Could you check a few things on this model? Use its own coordinates, in mm. Round coordinates to 2 decimals unless told otherwise and drop trailing zeros. Loops run counter-clockwise (first coordinate to the right, second up) from the corner with the lowest first, then second, coordinate; pieces in that order, holes last. Notation, with made-up numbers: (58.5, 5) - (99.5, 5) arc R23 ccw to (99.5, 34) - close; hole circle Ø6 at (-27, 67). An arc over 180 degrees is marked (long way). Use one line per item in the form item = value.
```python
from build123d import *

# Parameters (mm, degrees)
BOSS_EXTRUDE1_DEPTH = 1.5
SKETCH2_R           = 9
CUT_EXTRUDE3_DEPTH  = 1.5


with BuildPart() as part:
    # Sketch1 → Boss-Extrude1 (new body)
    with BuildSketch(Plane(origin=(0, 0, 0), x_dir=(1, 0, 0), z_dir=(0, 1, 0))):
        with BuildLine():
            Line((-97.5, 40), (97.5, 40))
            ThreePointArc((97.5, 40), (115.17766953, 32.67766953), (122.5, 15))
            Line((122.5, 15), (122.5, -15))
            ThreePointArc((122.5, -15), (115.17766953, -32.67766953), (97.5, -40))
            Line((97.5, -40), (-97.5, -40))
            ThreePointArc((-97.5, -40), (-115.17766953, -32.67766953), (-122.5, -15))
            Line((-122.5, -15), (-122.5, 15))
            ThreePointArc((-122.5, 15), (-115.17766953, 32.67766953), (-97.5, 40))
        make_face()
    extrude(amount=BOSS_EXTRUDE1_DEPTH)

    # Sketch2 → Cut-Extrude3 (cut)
    with BuildSketch(Plane(origin=(0, 1.5, 0), x_dir=(1, 0, 0), z_dir=(0, 1, 0))):
        with Locations(Location((75, 0, 0), (0, 0, 270))):
            Circle(SKETCH2_R)
        with Locations(Location((50, 0, 0), (0, 0, 270))):
            Circle(SKETCH2_R)
        with Locations(Location((25, 0, 0), (0, 0, 270))):
            Circle(SKETCH2_R)
        with Locations(Location((0, 0, 0), (0, 0, 270))):
            Circle(SKETCH2_R)
        with BuildLine():
            Line((99.15, -9), (122.5, -9))
            Line((122.5, -9), (122.5, 9))
            Line((122.5, 9), (99.15, 9))
            ThreePointArc((99.15, 9), (90.15, 0), (99.15, -9))
        make_face()
    extrude(amount=-CUT_EXTRUDE3_DEPTH, mode=Mode.SUBTRACT)


solid = part.part
```
1. If we section it at C-C, the plane y = 0.25: Write out the boundary of the cut face in (x, z).
Solution:
outline = (-122.5, -15) arc R25 ccw to (-97.5, -40) - (97.5, -40) arc R25 ccw to (122.5, -15) - (122.5, -9) - (99.15, -9) arc R9 cw to (99.15, 9) - (122.5, 9) - (122.5, 15) arc R25 ccw to (97.5, 40) - (-97.5, 40) arc R25 ccw to (-122.5, 15) - close; hole circle Ø18 at (0, 0); hole circle Ø18 at (25, 0); hole circle Ø18 at (50, 0); hole circle Ø18 at (75, 0)
2. If we section it at A-A, the plane x = 50: Write out the boundary of the cut face in (y, z), plus the area to 3 significant figures.
Solution:
outline = (0, -40) - (1.5, -40) - (1.5, -9) - (0, -9) - close; (0, 9) - (1.5, 9) - (1.5, 40) - (0, 40) - close
area = 93.0 mm^2
3. If we section it at B-B, the plane z = 0: Write out the boundary of the cut face in (x, y).
Solution:
outline = (-122.5, 0) - (-9, 0) - (-9, 1.5) - (-122.5, 1.5) - close; (9, 0) - (16, 0) - (16, 1.5) - (9, 1.5) - close; (34, 0) - (41, 0) - (41, 1.5) - (34, 1.5) - close; (59, 0) - (66, 0) - (66, 1.5) - (59, 1.5) - close; (84, 0) - (90.15, 0) - (90.15, 1.5) - (84, 1.5) - close
4. We'd pull the mould along Z, two halves only. Please class faces 1 (the face through (-115.371, 0.74, -32.482)), 2 (the face through (58.923, 0.76, -1.172)), 3 (the face through (-114.982, 0.74, 32.871)): +Z half, -Z half, draft (parallel to the pull), parting line (faces both ways), or undercut.
Solution:
face_1 = -Z half
face_2 = undercut
face_3 = +Z half
5. Please list where these lines run through material, in increasing order: line 1 along X through (y, z) = (1.1, 0); line 2 along X through (y, z) = (1, 7); line 3 along X through (y, z) = (0.25, -17.5).
Solution:
line_1 = -122.5 to -9, 9 to 16, 34 to 41, 59 to 66, 84 to 90.15
line_2 = -122.5 to -5.66, 5.66 to 19.34, 30.66 to 44.34, 55.66 to 69.34, 80.66 to 93.49
line_3 = -122.37 to 122.37
6. For P1, Ø23.5, axis at x = 0, z = 0, coming from the +Y side; P2, Ø0.8, axis at x = 113.5, y = 0.5, coming from the +Z side, each with a flat end and sliding along its axis, tell me the tip position at first contact or that it passes through.
Solution:
P1 = 1.5
P2 = 34.54
